from build123d import *

# Parameters (mm, degrees)
SKETCH1_R           = 1.25
BOSS_EXTRUDE1_DEPTH = 3.9
BOSS_EXTRUDE2_DEPTH = 8
SKETCH3_R           = 1.45181539
CUT_EXTRUDE1_DEPTH  = 4.8
SKETCH4_OUTSIDE_W   = 36.034
SKETCH4_OUTSIDE_H   = 36.72
SKETCH4_OUTSIDE_R   = 2.25
CUT_EXTRUDE2_DEPTH  = 13.387300307
CUT_EXTRUDE2_DRAFT  = -45
SKETCH5_OUTSIDE_W   = 28.676
SKETCH5_OUTSIDE_H   = 29.362
SKETCH5_OUTSIDE_R   = 2.25
CUT_EXTRUDE3_DEPTH  = 9.708341341
CUT_EXTRUDE3_DRAFT  = -45
CHAMFER1_SIZE       = 0.3
CHAMFER1_SIZE2      = 0.357526078


with BuildPart() as part:
    # Sketch1 → Boss-Extrude1 (new body)
    with BuildSketch(Plane(origin=(0, 0, 0), x_dir=(1, 0, 0), z_dir=(0, 1, 0))):
        with Locations(Location((0, 0, 0), (0, 0, 270))):
            Circle(SKETCH1_R)
    extrude(amount=BOSS_EXTRUDE1_DEPTH)

    # Sketch2 → Boss-Extrude2 (add)
    with BuildSketch(Plane(origin=(0, 3.9, 0), x_dir=(1, 0, 0), z_dir=(0, 1, 0))):
        Polygon((2.244901907, -1.307828516), (2.255063672, 1.290227823), (0.010161765, 2.598056339), (-2.244901907, 1.307828516), (-2.255063672, -1.290227823), (-0.010161765, -2.598056339), align=None)
    extrude(amount=BOSS_EXTRUDE2_DEPTH)

    # Sketch3 → Cut-Extrude1 (cut)
    with BuildSketch(Plane(origin=(0, 11.9, 0), x_dir=(1, 0, 0), z_dir=(0, 1, 0))):
        with Locations(Location((0, 0, 0), (0, 0, 270))):
            Circle(SKETCH3_R)
    extrude(amount=-CUT_EXTRUDE1_DEPTH, mode=Mode.SUBTRACT)


with BuildPart() as cut_extrude2_tool:
    # Sketch4 outside → Cut-Extrude2 (with draft: the straight prism first)
    with BuildSketch(Plane(origin=(0, 11.9, 0), x_dir=(1, 0, 0), z_dir=(0, 1, 0))):
        Rectangle(SKETCH4_OUTSIDE_W, SKETCH4_OUTSIDE_H)
        Circle(SKETCH4_OUTSIDE_R, mode=Mode.SUBTRACT)
    extrude(amount=-CUT_EXTRUDE2_DEPTH)
    # Cut-Extrude2: the draft: its side faces are tilted about the plane it starts from
    cut_extrude2_sides = [cut_extrude2_tool.faces().sort_by_distance(p)[0] for p in [
        (0, 5.206349846, 18.36),
        (18.017, 5.206349846, 0),
        (0, 5.206349846, -18.36),
        (-18.017, 5.206349846, 0),
        (-2.25, 5.206349846, 0),
    ]]
    draft(cut_extrude2_sides, Plane(origin=(0, 11.9, 0), x_dir=(1, 0, 0), z_dir=(0, 1, 0)), CUT_EXTRUDE2_DRAFT)


with BuildPart() as part_1:
    add(part.part)

    # Cut-Extrude2: cut by cut_extrude2_tool
    add(cut_extrude2_tool.part, mode=Mode.SUBTRACT)


with BuildPart() as cut_extrude3_tool:
    # Sketch5 outside → Cut-Extrude3 (with draft: the straight prism first)
    with BuildSketch(Plane.XZ.offset(-3.9)):
        Rectangle(SKETCH5_OUTSIDE_W, SKETCH5_OUTSIDE_H)
        Circle(SKETCH5_OUTSIDE_R, mode=Mode.SUBTRACT)
    extrude(amount=-CUT_EXTRUDE3_DEPTH)
    # Cut-Extrude3: the draft: its side faces are tilted about the plane it starts from
    cut_extrude3_sides = [cut_extrude3_tool.faces().sort_by_distance(p)[0] for p in [
        (0, 8.75417067, -14.681),
        (14.338, 8.75417067, 0),
        (0, 8.75417067, 14.681),
        (-14.338, 8.75417067, 0),
        (-2.25, 8.75417067, 0),
    ]]
    draft(cut_extrude3_sides, Plane.XZ.offset(-3.9), CUT_EXTRUDE3_DRAFT)


with BuildPart() as part_2:
    add(part_1.part)

    # Cut-Extrude3: cut by cut_extrude3_tool
    add(cut_extrude3_tool.part, mode=Mode.SUBTRACT)

    # Chamfer1
    chamfer1_edges = [part_2.edges().sort_by_distance(p)[0] for p in [
        (0, 0, -1.25),
    ]]
    chamfer1_side = [part_2.faces().sort_by_distance(p)[0] for p in [
        (0, 0, 0),
    ]]
    chamfer(chamfer1_edges, length=CHAMFER1_SIZE, length2=CHAMFER1_SIZE2, reference=chamfer1_side[0])


solid = part_2.part
Here's how the part is built. I have some questions about the finished solid (model axes, mm). A direction names the side the tool comes from. Coordinates: 2 decimals unless noted, no trailing zeros. Write each loop counter-clockwise with the first axis right and the second up, starting at its lowest first coordinate (ties: lowest second). Pieces come first, ordered by that corner, then holes.
Item 1: Will this pin go through, and if not, where does the flat tip stop? pin 1 (1.5 mm diameter, centred on x = 0.5, z = 0, fed in from +Y).
Item 2: If I drill on line 1 (X direction, y = 10.8, z = 0); line 2 (Y direction, x = -0.9, z = -2); line 3 (Z direction, x = 0.15, y = 7.25), over which ranges is the centre line in solid material (lowest first)?
Item 3: I want a section at B-B on y = 6. Write out the boundary of the cut face in (x, z).
Item 4: On a 3-axis mill with a long thin cutter (end or side, diameter ignored), from which of +Z, -Z, +X, -X, +Y, -Y can I reach the whole of each face in a straight line? I mean faces 4 (the flat face through (0, 7.1, 0)), 5 (the cylindrical face through (-1.22, 2.1, -0.27)), 6 (the flat face through (1.102, 7.844, 1.962)). Say none if no direction works.
Item 5: If we mould it in two halves opening along Z, with no side actions, what happens to faces 1 (the cylindrical face through (-1.42, 9.53, -0.31)), 2 (the conical face through (-2.05, 4.02, -1.19)), 3 (the flat face through (1, 3.9, 1))? For each: +Z half, -Z half, draft (parallel to the pull), parting line (faces both ways), or undercut.
Item 6: I want a section at A-A on y = 9.75. Write out the boundary of the cut face in (x, z), and give its area (3 significant figures).
Item 7: I want a section at C-C on y = 3.5. Write out the boundary of the cut face in (x, z), and give its area (3 significant figures).
Findings below:
1. pin 1: stops at y = 7.1
2. line 1: x = -2.25 to -1.45, 1.45 to 2.25
2. line 2: y = 3.9 to 11.9
2. line 3: z = -2.52 to -1.44, 1.44 to 2.51
3. outline: (-2.26, 1.29) - (-2.24, -1.31) - (0.01, -2.6) - (2.26, -1.29) - (2.24, 1.31) - (-0.01, 2.6) - close
4. face 4: +Y
4. face 5: -Y
4. face 6: +Z, +X, +Y, -Y
5. face 1: undercut
5. face 2: -Z half
5. face 3: draft
6. outline: (-2.26, 1.29) - (-2.24, -1.31) - (0.01, -2.6) - (2.26, -1.29) - (2.24, 1.31) - (-0.01, 2.6) - close; hole circle Ø2.9 at (0, 0)
6. area: 10.9 mm2
7. outline: circle Ø2.5 at (0, 0)
7. area: 4.91 mm2
